Design review of the part built by this model. Coordinates are the model's own, in mm. A direction names the side the tool comes from. Give positions to 0.01 mm unless a question says otherwise; leave off trailing zeros. Order: outer loops, then holes, each group sorted by start corner. A loop starts at its lowest first (then second) coordinate and runs counter-clockwise, first axis right, second up. Notation, with made-up numbers: M -37,-11 L 17,-11 A13 ccw 17,-2 Z; hole C 19.25,4 d2. An arc over 180 degrees is marked long. Answer as a JSON object with one key per item and string values.
from build123d import *

# Parameters (mm, degrees)
SKETCH1_R           = 10
BOSS_EXTRUDE1_DEPTH = 7
SKETCH2_R           = 10
SKETCH2_R_2         = 7.5
CUT_EXTRUDE2_DEPTH  = 5
CUT_EXTRUDE3_REACH  = 21.9
SKETCH3_R           = 2.5


with BuildPart() as part:
    # Sketch1 → Boss-Extrude1 (new, symmetric)
    with BuildSketch(Plane.XY):
        Circle(SKETCH1_R)
    extrude(amount=BOSS_EXTRUDE1_DEPTH, both=True)

    # Sketch2 → Cut-Extrude2 (cut, symmetric)
    with BuildSketch(Plane.XY):
        Circle(SKETCH2_R)
        Circle(SKETCH2_R_2, mode=Mode.SUBTRACT)
    extrude(amount=CUT_EXTRUDE2_DEPTH, both=True, mode=Mode.SUBTRACT)

    # Sketch3 → Cut-Extrude3 (cut, up to next)
    with BuildSketch(Plane.XY.offset(7), mode=Mode.PRIVATE) as cut_extrude3_sk1:
        Circle(SKETCH3_R)
    cut_extrude3_tool1 = extrude(cut_extrude3_sk1.sketch, amount=-CUT_EXTRUDE3_REACH, mode=Mode.PRIVATE) & part.part
    add(cut_extrude3_tool1.solids().sort_by_distance((0, 0, 7))[0], mode=Mode.SUBTRACT)


solid = part.part
(1) We need section A-A (x = 0). Write out the cut boundary in (y, z).
Checked values:
{"outline": "M -10,-7 L -2.5,-7 L -2.5,7 L -10,7 L -10,5 L -7.5,5 L -7.5,-5 L -10,-5 Z; M 2.5,-7 L 10,-7 L 10,-5 L 7.5,-5 L 7.5,5 L 10,5 L 10,7 L 2.5,7 Z"}
(2) We need section B-B (y = 8.5). Write out the cut boundary in (x, z).
Checked values:
{"outline": "M -5.27,-7 L 5.27,-7 L 5.27,-5 L -5.27,-5 Z; M -5.27,5 L 5.27,5 L 5.27,7 L -5.27,7 Z"}
(3) To check wall thickness, follow L1, parallel to Y at x = 0, z = -3.25; L2, parallel to Z at x = -5.25, y = 7.25; L3, parallel to X at y = 1.75, z = 3.5. State the ranges of each line that lie inside material, in increasing order. Write a range as from..to.
Checked values:
{"L1": "y = -7.5..-2.5, 2.5..7.5", "L2": "z = -7..-5, 5..7", "L3": "x = -7.29..-1.79, 1.79..7.29"}
(4) Insertion check: pin 1 (6 mm diameter, centred on y = -2, z = -1.5, fed in from +X); pin 2 (2 mm diameter, centred on x = -4, z = -2, fed in from +Y); pin 3 (5 mm diameter, centred on x = 5, z = -5.5, fed in from -Y). Each pin has a flat end and moves straight along its axis. Give the tip position at first contact, or say it passes through.
Checked values:
{"pin 1": "stops at x = 7.5", "pin 2": "stops at y = 6.87", "pin 3": "stops at y = -9.68"}
(5) Tool access review of faces 4 (the flat face through (4, 7, 5)), 5 (the flat face through (2, -2, 7)): name each direction out of +Z, -Z, +X, -X, +Y, -Y from which nothing blocks a thin tool from reaching the whole face with its end or side.
Checked values:
{"face 4": "none", "face 5": "+Z, +X, -X, +Y, -Y"}
(6) Draft analysis for pull direction Y (two halves, no side actions). For faces 1 (the flat face through (4, 7, -5)), 2 (the cylindrical face through (-0.54, -2.44, 0.1)), 3 (the cylindrical face through (-7.493, 0.33, -0.07)), state which applies: +Y half, -Y half, draft (parallel to the pull), parting line (faces both ways), or undercut.
Checked values:
{"face 1": "draft", "face 2": "undercut", "face 3": "parting line"}
(7) We need section D-D (x = 7). Write out the cut boundary in (y, z), plus the area to 3 significant figures.
Checked values:
{"outline": "M -7.14,-7 L 7.14,-7 L 7.14,-5 L 2.69,-5 L 2.69,5 L 7.14,5 L 7.14,7 L -7.14,7 L -7.14,5 L -2.69,5 L -2.69,-5 L -7.14,-5 Z", "area": "111 mm^2"}
(8) We need section C-C (z = 2.5). Write out the cut boundary in (x, y), plus the area to 3 significant figures.
Checked values:
{"outline": "C 0,0 d15; hole C 0,0 d5", "area": "157 mm^2"}
